CAD build for the part. Positions are in the model's coordinates, mm. A direction names the side the tool comes from. Round coordinates to 2 decimals unless told otherwise and drop trailing zeros.
from build123d import *

# Parameters (mm, degrees)
F1_DEPTH = 304.8


with BuildPart() as f1:
    # F0 (on Front) → F1 (new body)
    with BuildSketch(Plane.XZ):
        Polygon((-100.0125, 33.3248), (-100.0125, 0), (100.0125, 0), (100.0125, 33.3248), (98.4885, 33.3248), (98.4885, 7.9248), (92.07246, 7.9248), (92.07246, 33.3248), (90.54846, 33.3248), (90.54846, 7.9248), (84.13242, 7.9248), (84.13242, 33.3248), (82.60842, 33.3248), (82.60842, 7.9248), (76.19238, 7.9248), (76.19238, 33.3248), (74.66838, 33.3248), (74.66838, 7.9248), (68.25234, 7.9248), (68.25234, 33.3248), (66.72834, 33.3248), (66.72834, 7.9248), (60.3123, 7.9248), (60.3123, 33.3248), (58.7883, 33.3248), (58.7883, 7.9248), (52.37226, 7.9248), (52.37226, 33.3248), (50.84826, 33.3248), (50.84826, 7.9248), (44.43222, 7.9248), (44.43222, 33.3248), (42.90822, 33.3248), (42.90822, 7.9248), (36.49218, 7.9248), (36.49218, 33.3248), (34.96818, 33.3248), (34.96818, 7.9248), (28.55214, 7.9248), (28.55214, 33.3248), (27.02814, 33.3248), (27.02814, 7.9248), (20.6121, 7.9248), (20.6121, 33.3248), (19.0881, 33.3248), (19.0881, 7.9248), (12.67206, 7.9248), (12.67206, 33.3248), (11.14806, 33.3248), (11.14806, 7.9248), (4.73202, 7.9248), (4.73202, 33.3248), (3.20802, 33.3248), (3.20802, 7.9248), (-3.20802, 7.9248), (-3.20802, 33.3248), (-4.73202, 33.3248), (-4.73202, 7.9248), (-11.14806, 7.9248), (-11.14806, 33.3248), (-12.67206, 33.3248), (-12.67206, 7.9248), (-19.0881, 7.9248), (-19.0881, 33.3248), (-20.6121, 33.3248), (-20.6121, 7.9248), (-27.02814, 7.9248), (-27.02814, 33.3248), (-28.55214, 33.3248), (-28.55214, 7.9248), (-34.96818, 7.9248), (-34.96818, 33.3248), (-36.49218, 33.3248), (-36.49218, 7.9248), (-42.90822, 7.9248), (-42.90822, 33.3248), (-44.43222, 33.3248), (-44.43222, 7.9248), (-50.84826, 7.9248), (-50.84826, 33.3248), (-52.37226, 33.3248), (-52.37226, 7.9248), (-58.7883, 7.9248), (-58.7883, 33.3248), (-60.3123, 33.3248), (-60.3123, 7.9248), (-66.72834, 7.9248), (-66.72834, 33.3248), (-68.25234, 33.3248), (-68.25234, 7.9248), (-74.66838, 7.9248), (-74.66838, 33.3248), (-76.19238, 33.3248), (-76.19238, 7.9248), (-82.60842, 7.9248), (-82.60842, 33.3248), (-84.13242, 33.3248), (-84.13242, 7.9248), (-90.54846, 7.9248), (-90.54846, 33.3248), (-92.07246, 33.3248), (-92.07246, 7.9248), (-98.4885, 7.9248), (-98.4885, 33.3248), align=None)
    extrude(amount=F1_DEPTH)


solid = f1.part
Item 1: Cut at A-A (z = 18). State how many separate pieces and enclosed holes the cut face has, plus the area to 3 significant figures.
Verdict:
separate pieces: 26
enclosed holes: 0
area: 12,100 mm2
Item 2: Flat gauge pins, fed straight in: P1, Ø5, axis at x = 87.5, y = -166, coming from the +Z side; P2, Ø4, axis at x = -17, z = 11.5, coming from the +Y side. Where does each tip first touch, or does it go through?
Verdict:
P1: stops at z = 7.92
P2: passes through
Item 3: 3-axis set-ups, long thin cutter, end or side, ignore diameter. For faces 1 (the flat face through (4.732, -150, 20)), 2 (the flat face through (-1, -150, 0)): which of +Z, -Z, +X, -X, +Y, -Y reach the whole face in a straight line?
Verdict:
face 1: +Z, +Y, -Y
face 2: -Z, +X, -X, +Y, -Y
Item 4: Wall check: L1, parallel to Z at x = -25, y = -94. Give the ranges that are in metal, low to high.
Verdict:
L1: z = 0 to 7.92
